from build123d import *

# Parameters (mm, degrees)
SKETCH1_R           = 6
BOSS_EXTRUDE1_DEPTH = 19
SKETCH2_R           = 12
CUT_EXTRUDE1_DEPTH  = 99.620484688


with BuildPart() as part:
    # Sketch1 → Boss-Extrude1 (new, symmetric)
    with BuildSketch(Plane.XY):
        with BuildLine():
            Line((0, 19), (70, 19))
            ThreePointArc((70, 19), (89, 0), (70, -19))
            Line((70, -19), (0, -19))
            ThreePointArc((0, -19), (-19, 0), (0, 19))
        make_face()
        Circle(SKETCH1_R, mode=Mode.SUBTRACT)
        with Locations((70, 0)):
            Circle(SKETCH1_R, mode=Mode.SUBTRACT)
    extrude(amount=BOSS_EXTRUDE1_DEPTH, both=True)

    # Sketch2 → Cut-Extrude1 (cut, through all)
    with BuildSketch(Plane.XZ.offset(19)):
        with Locations(Location((35, 0, 0), (0, 0, 270))):
            Circle(SKETCH2_R)
    extrude(amount=-CUT_EXTRUDE1_DEPTH, mode=Mode.SUBTRACT)


solid = part.part
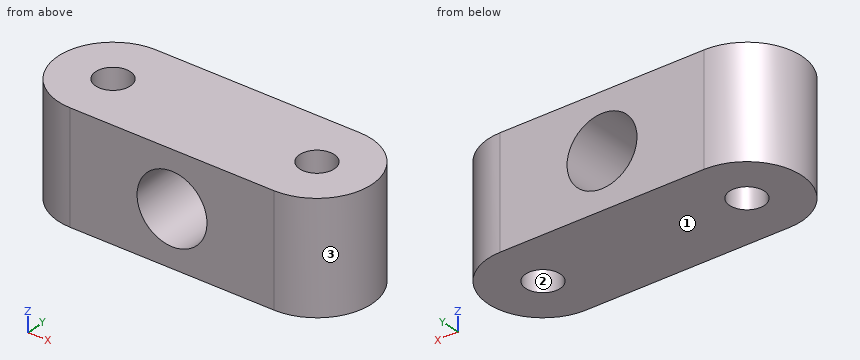
Design review of the part built by this model. Coordinates are the model's own, in mm. Face numbers are marked on the shaded views. Round coordinates to 2 decimals unless told otherwise and drop trailing zeros. Loops run counter-clockwise (first coordinate to the right, second up) from the corner with the lowest first, then second, coordinate; pieces in that order, holes last. Notation, with made-up numbers: (-5.5, 17) -> (49.5, 17) arc R13 ccw to (49.5, 27) -> close; hole circle Ø4 at (-2.5, 83.5). An arc over 180 degrees is marked (long way). Use one line per item in the form item = value. Start each with the question number.
Q1. We need section D-D on z = -16. Give the boundary of the cut face in (x, y), then the cut area to 3 significant figures.
Q2. Wall thickness on line 1 along Y through (x, z) = (70, 3); line 2 along X through (y, z) = (1.5, 4.5); line 3 along X through (y, z) = (2.5, 3.5): over which ranges is each line inside the solid? List them lowest first. Write a range as [from, to].
Q3. We need section C-C on z = 0. Give the boundary of the cut face in (x, y), then the cut area to 3 significant figures.
Q4. We need section A-A on y = 0. Give the boundary of the cut face in (x, z), then the cut area to 3 significant figures.
Q5. For pin 1 Ø6 at (y, z) = (5.5, -9.5) entering from +X; pin 2 Ø3 at (y, z) = (6.5, -10.5) entering from +X; pin 3 Ø4 at (y, z) = (-9.5, -10) entering from -X, all flat-tipped, find the tip position at first contact; note any pin that passes through.
Q6. We need section B-B on x = 35. Give the boundary of the cut face in (y, z), then the cut area to 3 significant figures.
Q7. Draft analysis for pull direction X (two halves, no side actions). For the marked faces 1, 2 and 3, state which applies: +X half, -X half, draft (parallel to the pull), parting line (faces both ways), or undercut.
Calculated:
q1.outline = (0, -19) -> (70, -19) arc R19 ccw to (70, 19) -> (0, 19) arc R19 ccw to start; hole circle Ø12 at (0, 0); hole circle Ø12 at (70, 0)
q1.area = 3,570 mm²
q2.line_1 = [-19, -6], [6, 19]
q2.line_2 = [-18.94, -5.81], [5.81, 23.88], [46.12, 64.19], [75.81, 88.94]
q2.line_3 = [-18.83, -5.45], [5.45, 23.52], [46.48, 64.55], [75.45, 88.83]
q3.outline = (0, -19) -> (23, -19) -> (23, 19) -> (0, 19) arc R19 ccw to start; (47, -19) -> (70, -19) arc R19 ccw to (70, 19) -> (47, 19) -> close; hole circle Ø12 at (0, 0); hole circle Ø12 at (70, 0)
q3.area = 2,660 mm²
q4.outline = (-19, -19) -> (-6, -19) -> (-6, 19) -> (-19, 19) -> close; (6, -19) -> (64, -19) -> (64, 19) -> (6, 19) -> close; (76, -19) -> (89, -19) -> (89, 19) -> (76, 19) -> close; hole circle Ø24 at (35, 0)
q4.area = 2,740 mm²
q5.pin_1 = 88.83
q5.pin_2 = 88.33
q5.pin_3 = -17.46
q6.outline = (-19, -19) -> (19, -19) -> (19, -12) -> (-19, -12) -> close; (-19, 12) -> (19, 12) -> (19, 19) -> (-19, 19) -> close
q6.area = 532 mm²
q7.face_1 = draft
q7.face_2 = undercut
q7.face_3 = +X half
